Read the model definition and answer for the solid it produces. Units are mm, in the model's axes. Face numbers are marked on the shaded views. A direction names the side the tool comes from. Give positions to 0.01 mm unless a question says otherwise; leave off trailing zeros. Order: outer loops, then holes, each group sorted by start corner. A loop starts at its lowest first (then second) coordinate and runs counter-clockwise, first axis right, second up. Notation, with made-up numbers: (-4, 67.5) - (8, 67.5) arc R23 cw to (8, 79.5) - close; hole circle Ø3 at (51.25, 6.25). An arc over 180 degrees is marked (long way). Use a Markdown table: item, result. Add a question column.
1. A cutting plane is placed at B-B on y = 16.75. Determine the outline of the cut face in (x, z).
2. A cutting plane is placed at C-C on x = -17.5. Determine the outline of the cut face in (y, z).
3. A cutting plane is placed at A-A on x = -26. Determine the outline of the cut face in (y, z).
4. For a pull along Z with two mould halves and no side action, classify the marked faces 1, 2 and 3 as released by +Z, released by -Z, zero draft, split by the parting line, or undercut.
5. Consider L1, parallel to Z at x = -15, y = 4.5; L2, parallel to X at y = 13.75, z = 40.5; L3, parallel to Z at x = -31.5, y = 12.25. Determine where each line is inside the solid, lowest interval first.
6. Which of the six approach directions +Z, -Z, +X, -X, +Y, -Y give full straight-line access (tool end or side, diameter ignored) to the marked faces 4, 5 and 6?
7. A cutting plane is placed at D-D on z = 29. Determine the outline of the cut face in (x, y), and give its area (3 significant figures).
8. Flat-ended cylindrical pins translate along their axes: P1, Ø10, axis at y = 9, z = 31, coming from the -X side; P2, Ø3, axis at y = 5.25, z = -27.53, coming from the +X side; P3, Ø2, axis at y = 8.5, z = -10, coming from the -X side; P4, Ø3, axis at y = 5.5, z = 42, coming from the -X side. Find the tip coordinate at first contact, or state that the pin passes through.
```python
from build123d import *

# Parameters (mm, degrees)
BOSS_EXTRUDE1_DEPTH = 18
SKETCH2_R           = 1.75
CUT_EXTRUDE1_DEPTH  = 33.5
CUT_EXTRUDE2_DEPTH  = 1
CUT_EXTRUDE3_DEPTH  = 5


with BuildPart() as part:
    # Sketch1 → Boss-Extrude1 (new body)
    with BuildSketch(Plane(origin=(0, 0, 0), x_dir=(1, 0, 0), z_dir=(0, 1, 0))):
        with BuildLine():
            Line((-11.998275301, 32.528571429), (-29.498275301, 32.528571429))
            Line((-29.498275301, 32.528571429), (-29.498275301, 19.914699304))
            ThreePointArc((-29.498275301, 19.914699304), (-21.114218589, 23.723916882), (-11.998275301, 25.028571429))
            Line((-11.998275301, 25.028571429), (-11.998275301, 32.528571429))
        make_face()
        with BuildLine():
            ThreePointArc((-11.998275301, 25.028571429), (-21.114218589, 23.723916882), (-29.498275301, 19.914699304))
            ThreePointArc((-29.498275301, 19.914699304), (-44.498275301, -7.471428571), (-29.498275301, -34.857556447))
            ThreePointArc((-29.498275301, -34.857556447), (-21.114218589, -38.666774025), (-11.998275301, -39.971428571))
            Line((-11.998275301, -39.971428571), (-11.998275301, -32.971428571))
            ThreePointArc((-11.998275301, -32.971428571), (-37.498275301, -7.471428571), (-11.998275301, 18.028571429))
            Line((-11.998275301, 18.028571429), (-11.998275301, 25.028571429))
        make_face()
        with BuildLine():
            Line((-29.498275301, -34.857556447), (-29.498275301, -47.471428571))
            Line((-29.498275301, -47.471428571), (-11.998275301, -47.471428571))
            Line((-11.998275301, -47.471428571), (-11.998275301, -39.971428571))
            ThreePointArc((-11.998275301, -39.971428571), (-21.114218589, -38.666774025), (-29.498275301, -34.857556447))
        make_face()
    extrude(amount=BOSS_EXTRUDE1_DEPTH)

    # Sketch2 → Cut-Extrude1 (cut, through all)
    with BuildSketch(Plane(origin=(-11.998275301, 0, 0), x_dir=(0, 0, -1), z_dir=(1, 0, 0))):
        with Locations((-42.471428571, 5.25)):
            Circle(SKETCH2_R)
        with Locations((27.528571429, 5.25)):
            Circle(SKETCH2_R)
    extrude(amount=-CUT_EXTRUDE1_DEPTH, mode=Mode.SUBTRACT)

    # Sketch3 → Cut-Extrude2 (cut)
    with BuildSketch(Plane(origin=(-11.998275301, 0, 0), x_dir=(0, 0, -1), z_dir=(1, 0, 0))):
        Polygon((-42.326802517, 14.778828324), (-39.748811064, 14.778828324), (-39.748811064, 13.829042), (-41.377016192, 13.829042), (-41.377016192, 12.811413795), (-39.748811064, 12.811413795), (-39.748811064, 11.86162747), (-41.377016192, 11.86162747), (-41.377016192, 9.487161658), (-42.326802517, 9.487161658), align=None)
        with BuildLine():
            Line((-37.488828425, 9.351477897), (-38.330491753, 9.775489649))
            Line((-38.330491753, 9.775489649), (-37.408266192, 11.590259948))
            add(Edge.make_bspline(
                [(-37.408266192, 11.590259948), (-37.462753396, 11.591648755), (-37.569724958, 11.594375318), (-37.727232239, 11.617033031), (-37.87785266, 11.655711194), (-38.023361539, 11.707201572), (-38.161746535, 11.77622976), (-38.294685676, 11.858611279), (-38.420338635, 11.95759149), (-38.539294546, 12.068849341), (-38.647905095, 12.191825278), (-38.742176754, 12.324083818), (-38.824345348, 12.462269948), (-38.888244154, 12.60950332), (-38.939568, 12.76303987), (-38.977067789, 12.92367432), (-38.998111679, 13.092111431), (-39.00105302, 13.206747887), (-39.00255038, 13.265106369)],
                knots=[0, 0, 0, 0, 0.000163413, 0.000320819, 0.000476106, 0.000629341, 0.000782939, 0.000939124, 0.001097732, 0.001261968, 0.001427204, 0.001589, 0.001748625, 0.001908563, 0.002069464, 0.002233772, 0.002402593, 0.002577655, 0.002577655, 0.002577655, 0.002577655], degree=3))
            add(Edge.make_bspline(
                [(-39.00255038, 13.265106369), (-39.001161497, 13.321713522), (-38.99842473, 13.433256746), (-38.975695616, 13.5969659), (-38.938289378, 13.754150604), (-38.88696936, 13.904784157), (-38.818649356, 14.047850808), (-38.738682529, 14.185590652), (-38.640926713, 14.315153998), (-38.530495897, 14.437101726), (-38.409635229, 14.548662366), (-38.281412206, 14.646751431), (-38.146409838, 14.728744465), (-38.006363041, 14.797603487), (-37.858740367, 14.849050664), (-37.705675127, 14.887867179), (-37.546027089, 14.910269855), (-37.43766133, 14.913086693), (-37.382825487, 14.914512085)],
                knots=[0, 0, 0, 0, 0.000169767, 0.000334522, 0.000494702, 0.000653936, 0.000810896, 0.000969607, 0.001130944, 0.0012968, 0.001462589, 0.001623717, 0.001780246, 0.001935749, 0.002090981, 0.002248323, 0.002408879, 0.002573351, 0.002573351, 0.002573351, 0.002573351], degree=3))
            add(Edge.make_bspline(
                [(-37.382825487, 14.914512085), (-37.32548798, 14.913331855), (-37.212741531, 14.911011091), (-37.047695871, 14.885402378), (-36.889786863, 14.846113929), (-36.738372898, 14.792752199), (-36.595333717, 14.720329287), (-36.459472442, 14.633529923), (-36.331240989, 14.530433614), (-36.212016472, 14.414011914), (-36.103583105, 14.287381533), (-36.007470418, 14.154830073), (-35.92673168, 14.016616709), (-35.860601716, 13.873974949), (-35.809086806, 13.726681326), (-35.773676871, 13.574526911), (-35.750168601, 13.417771894), (-35.747493829, 13.311480409), (-35.746140124, 13.257686164)],
                knots=[0, 0, 0, 0, 0.000171885, 0.000337989, 0.000499701, 0.000659639, 0.000818449, 0.000979588, 0.001142488, 0.001311152, 0.001478788, 0.001642063, 0.001801688, 0.0019582, 0.00211308, 0.00226889, 0.002426296, 0.002587592, 0.002587592, 0.002587592, 0.002587592], degree=3))
            add(Edge.make_bspline(
                [(-35.746140124, 13.257686164), (-35.746878854, 13.21665857), (-35.748366821, 13.134019773), (-35.762997646, 13.010093938), (-35.785195556, 12.885824631), (-35.810960929, 12.781344964), (-35.837972338, 12.693274952), (-35.864257515, 12.618563879), (-35.897982171, 12.535620561), (-35.935639121, 12.443889047), (-35.9792503, 12.343771591), (-36.029719907, 12.235746792), (-36.083997697, 12.118212537), (-36.124005786, 12.037844215), (-36.144711171, 11.996251201)],
                knots=[0, 0, 0, 0, 0.000123036, 0.000247823, 0.000373829, 0.000501605, 0.000570344, 0.000650135, 0.000739108, 0.000838914, 0.000947623, 0.001066672, 0.001196607, 0.001335984, 0.001335984, 0.001335984, 0.001335984], degree=3))
            Line((-36.144711171, 11.996251201), (-37.488828425, 9.351477897))
        make_face()
        with BuildLine():
            add(Edge.make_bspline(
                [(-37.3616249, 12.472204393), (-37.316115096, 12.474883687), (-37.227199244, 12.480118421), (-37.099477536, 12.520594498), (-36.985173101, 12.58986006), (-36.883860931, 12.68188028), (-36.800139654, 12.794149159), (-36.739268808, 12.921957298), (-36.70177424, 13.062657931), (-36.697913156, 13.160632443), (-36.695926449, 13.211044871)],
                knots=[0, 0, 0, 0, 0.000136382, 0.000266459, 0.00039717, 0.000534504, 0.00067464, 0.000814508, 0.000956947, 0.001107922, 0.001107922, 0.001107922, 0.001107922], degree=3))
            add(Edge.make_bspline(
                [(-36.695926449, 13.211044871), (-36.698319221, 13.262505994), (-36.702973734, 13.362610164), (-36.740827484, 13.506688151), (-36.805511929, 13.636926106), (-36.893511418, 13.750138756), (-36.996249672, 13.84488328), (-37.111136974, 13.914091604), (-37.23538362, 13.956887813), (-37.321366646, 13.962095071), (-37.364804988, 13.96472576)],
                knots=[0, 0, 0, 0, 0.00015423, 0.000300014, 0.00044318, 0.000587566, 0.000727895, 0.000860059, 0.000987439, 0.001117495, 0.001117495, 0.001117495, 0.001117495], degree=3))
            add(Edge.make_bspline(
                [(-37.364804988, 13.96472576), (-37.410716877, 13.962161178), (-37.500864495, 13.95712564), (-37.630172561, 13.914432203), (-37.749374298, 13.84655291), (-37.853470467, 13.751486921), (-37.943561709, 13.639765246), (-38.006384791, 13.50908768), (-38.046128852, 13.366015125), (-38.050512553, 13.265731436), (-38.052764056, 13.214224959)],
                knots=[0, 0, 0, 0, 0.000137436, 0.000269855, 0.000404228, 0.000546134, 0.000690333, 0.00083208, 0.000978137, 0.001132367, 0.001132367, 0.001132367, 0.001132367], degree=3))
            add(Edge.make_bspline(
                [(-38.052764056, 13.214224959), (-38.050412222, 13.163452669), (-38.04583815, 13.064705867), (-38.007502778, 12.923207265), (-37.945058299, 12.794722755), (-37.859692241, 12.681568477), (-37.75454228, 12.589094862), (-37.635152594, 12.520567119), (-37.501976162, 12.48000867), (-37.409250814, 12.474852647), (-37.3616249, 12.472204393)],
                knots=[0, 0, 0, 0, 0.000152117, 0.000295852, 0.00043618, 0.000578438, 0.000718145, 0.000853439, 0.000988579, 0.00113129, 0.00113129, 0.00113129, 0.00113129], degree=3))
        make_face(mode=Mode.SUBTRACT)
    extrude(amount=-CUT_EXTRUDE2_DEPTH, mode=Mode.SUBTRACT)

    # Sketch4 → Cut-Extrude3 (cut)
    with BuildSketch(Plane.ZY.offset(29.498275301)):
        Polygon((-25.391799088, 2.901056132), (-24.425940196, 5.926027195), (-26.562712537, 8.274971063), (-29.665343769, 7.598943868), (-30.631202661, 4.573972805), (-28.49443032, 2.225028937), align=None)
        Polygon((44.716794169, 3.004634402), (45.538655018, 6.071860849), (43.293289421, 8.317226447), (40.226062974, 7.495365598), (39.404202124, 4.428139151), (41.649567722, 2.182773553), align=None)
    extrude(amount=-CUT_EXTRUDE3_DEPTH, mode=Mode.SUBTRACT)


solid = part.part
```
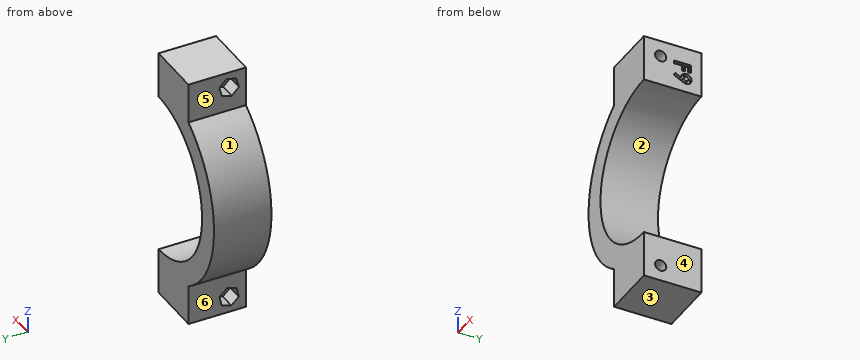
Output values:
| question | item | result |
|---|---|---|
| 1 | outline | (-29.5, -32.53) - (-12, -32.53) - (-12, -18.03) arc R25.5 cw to (-12, 32.97) - (-12, 47.47) - (-29.5, 47.47) - (-29.5, 34.86) arc R32.5 ccw to (-29.5, -19.91) - close |
| 2 | outline | (0, -32.53) - (18, -32.53) - (18, -17.43) - (0, -17.43) - close; (0, 32.37) - (18, 32.37) - (18, 47.47) - (0, 47.47) - close; hole circle Ø3.5 at (5.25, -27.53); hole circle Ø3.5 at (5.25, 42.47) |
| 3 | outline | (0, -32.53) - (18, -32.53) - (18, -13.84) - (0, -13.84) - close; (0, 28.78) - (18, 28.78) - (18, 47.47) - (0, 47.47) - close; hole (2.18, 41.65) - (4.43, 39.4) - (7.5, 40.23) - (8.32, 43.29) - (6.07, 45.54) - (3, 44.72) - close; hole (2.23, -28.49) - (4.57, -30.63) - (7.6, -29.67) - (8.27, -26.56) - (5.93, -24.43) - (2.9, -25.39) - close |
| 4 | face 1 | split by the parting line |
| 4 | face 2 | undercut |
| 4 | face 3 | released by -Z |
| 5 | L1 | -32.53 to -29.11, -25.95 to -17.85, 32.79 to 40.89, 44.05 to 47.47 |
| 5 | L2 | -29.5 to -12 |
| 5 | L3 | -18.53 to -8.96, 23.9 to 33.47 |
| 6 | face 4 | +Z, -Z, +X, +Y, -Y |
| 6 | face 5 | +Z, -X, +Y, -Y |
| 6 | face 6 | -Z, -X, +Y, -Y |
| 7 | outline | (-36.35, 0) - (-25.66, 0) - (-25.66, 18) - (-36.35, 18) - close |
| 7 | area | 192 mm² |
| 8 | P1 | x = -38.7 |
| 8 | P2 | through |
| 8 | P3 | x = -40.02 |
| 8 | P4 | x = -24.5 |
